Verification items for the finished model (mm, model axes). Round coordinates to 2 decimals unless told otherwise and drop trailing zeros. Order: outer loops, then holes, each group sorted by start corner. A loop starts at its lowest first (then second) coordinate and runs counter-clockwise, first axis right, second up. Notation, with made-up numbers: (32, -10) -> (51, -10) arc R26 cw to (51, 17) -> close; hole circle Ø10 at (41, -1). An arc over 180 degrees is marked (long way). Write item = value, one per line. Start each with the question number.
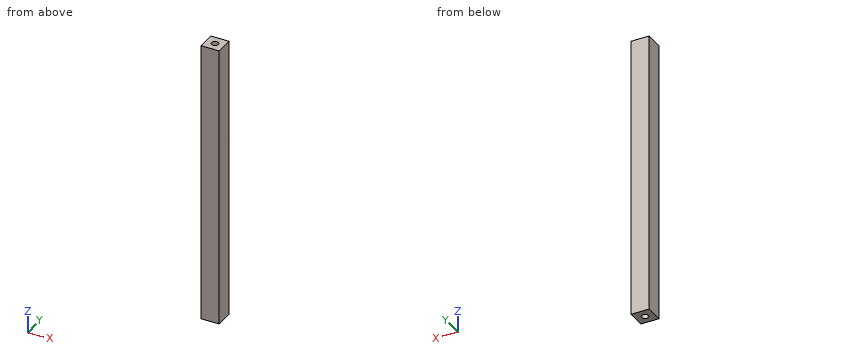
Autodesk Inventor part; units mm, degrees
ref_plane "YZ Plane" through (0, 0, 0) normal (1, 0, 0) x (0, 1, 0)
ref_plane "XZ Plane" through (0, 0, 0) normal (0, 1, 0) x (-1, 0, 0)
ref_plane "XY Plane" through (0, 0, 0) normal (0, 0, 1) x (1, 0, 0)
sketch "Sketch1" plane through (0, 0, 0) normal (0, 0, 1) x (1, 0, 0)
  line L0 (4, 4) -> (-4, 4)
  line L1 (-4, 4) -> (-4, -4)
  line L2 (-4, -4) -> (4, -4)
  line L3 (4, -4) -> (4, 4)
  line L4 (4, 4) -> (-4, -4) construction
  line L5 (-4, 4) -> (4, -4) construction
  point P0 (0, 0)
  dimension "d0" = 8
  dimension "d1" = 8
extrude "Extrusion1" add sketch "Sketch1" along normal blind 125
sketch "Sketch2" plane through (0, 0, 125) normal (0, 0, 1) x (1, 0, 0)
  circle A0 centre (0, 0) radius 1.5
  dimension "d4" = 3
extrude "Extrusion2" cut sketch "Sketch2" against normal blind 15
sketch "Sketch4" plane through (0, 0, 0) normal (0, 0, -1) x (-1, 0, 0)
  circle A0 centre (0, 0) radius 1.5
  circle A1 centre (0, 0) radius 1.5
  dimension "d11" = 3
extrude "Extrusion4" cut sketch "Sketch4" against normal blind 15
properties part number "bacaklar"
(1) Depth check by flat-ended pin: pin 1 (1.5 mm diameter, centred on x = -0.5, y = 0, fed in from -Z); pin 2 (0.9 mm diameter, centred on x = -0.5, y = 0, fed in from +Z). Enter the tip coordinate at first touch or a pass-through.
(2) Scan lines: line 1 along Y through (x, z) = (0, 113.75); line 2 along Z through (x, y) = (0.25, 0.75). Record each from-to range of solid material in increasing order. Write a range as from..to.
(3) Cross-section at A-A (x = 0). Enter the section's corners in (y, z), and give its area (3 significant figures).
Outcome:
q1.pin_1 = 15
q1.pin_2 = 110
q2.line_1 = -4..-1.5, 1.5..4
q2.line_2 = 15..110
q3.outline = (-4, 0) -> (-1.5, 0) -> (-1.5, 15) -> (1.5, 15) -> (1.5, 0) -> (4, 0) -> (4, 125) -> (1.5, 125) -> (1.5, 110) -> (-1.5, 110) -> (-1.5, 125) -> (-4, 125) -> close
q3.area = 910 mm^2
